Check sheet for the drawn part. Datum: minimum x, y, z corner. Units: mm. A direction names the side the tool comes from. Coordinates: 2 decimals unless noted, no trailing zeros. Write each loop counter-clockwise with the first axis right and the second up, starting at its lowest first coordinate (ties: lowest second). Pieces come first, ordered by that corner, then holes. Notation, with made-up numbers: (46.25, 32) -> (66.25, 32) arc R5 ccw to (66.25, 37) -> close; hole circle Ø6 at (-13, 50.25). An arc over 180 degrees is marked (long way). One line per question, with ' | ' between items.
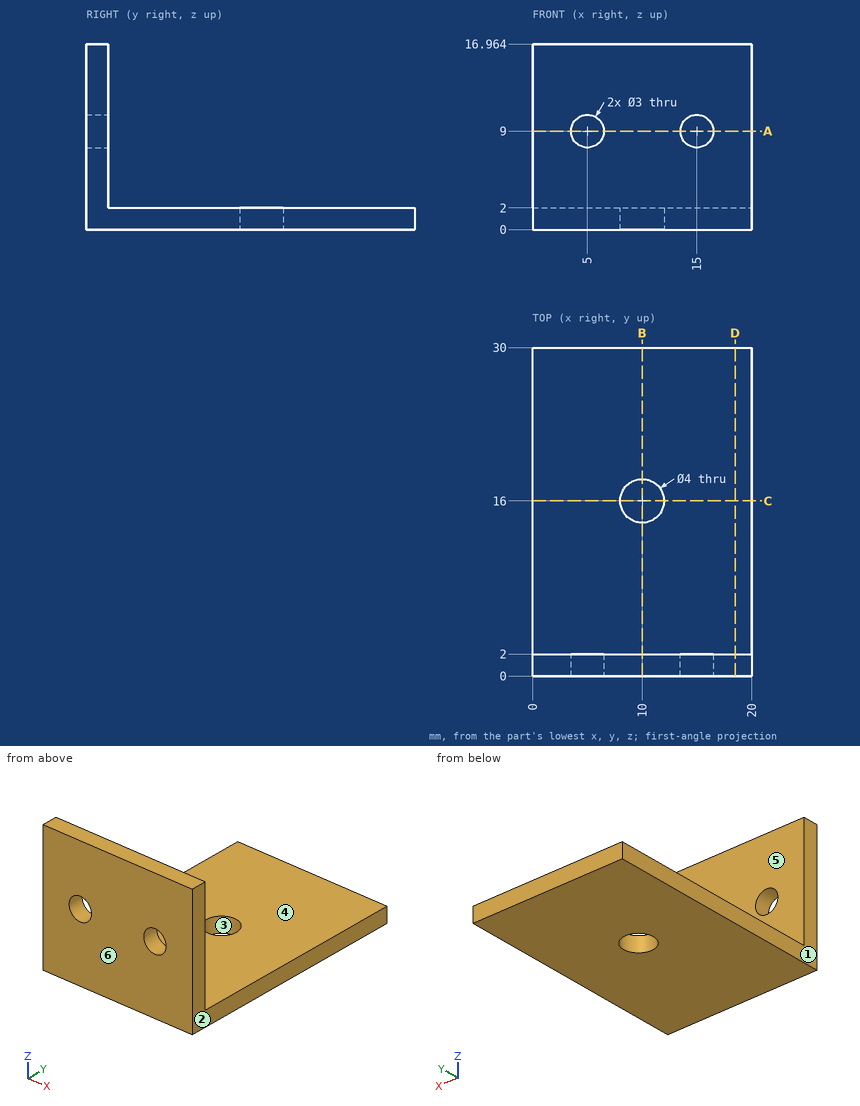
1. Cross-section at C-C on y = 16. Record the boundary of the cut face in (x, z).
Worked answers:
outline: (0, 0) -> (8, 0) -> (8, 2) -> (0, 2) -> close; (12, 0) -> (20, 0) -> (20, 2) -> (12, 2) -> close
2. Cross-section at A-A on z = 9. Record the boundary of the cut face in (x, y).
Worked answers:
outline: (0, 0) -> (3.5, 0) -> (3.5, 2) -> (0, 2) -> close; (6.5, 0) -> (13.5, 0) -> (13.5, 2) -> (6.5, 2) -> close; (16.5, 0) -> (20, 0) -> (20, 2) -> (16.5, 2) -> close
3. Cross-section at B-B on x = 10. Record the boundary of the cut face in (y, z).
Worked answers:
outline: (0, 0) -> (14, 0) -> (14, 2) -> (2, 2) -> (2, 16.96) -> (0, 16.96) -> close; (18, 0) -> (30, 0) -> (30, 2) -> (18, 2) -> close
4. Tool access check on the marked faces 5 and 6. Record the directions out of +Z, -Z, +X, -X, +Y, -Y that give a thin tool (end or side, any length) a straight path to the whole face; none if there is none.
Worked answers:
face 5: +Z, +X, -X, +Y | face 6: +Z, -Z, +X, -X, -Y
5. Mould release check, pull along X, two halves, no side actions. Record for the marked faces 1, 2, 3 and 4: released by +X, released by -X, zero draft, split by the parting line, or undercut.
Worked answers:
face 1: released by -X | face 2: released by +X | face 3: undercut | face 4: zero draft
6. Material ranges on line 1 (Z direction, x = 15, y = 0.55); line 2 (X direction, y = 0.5, z = 9); line 3 (Y direction, x = 10, z = 1.4), recorded low to high. Write a range as from..to.
Worked answers:
line 1: 0..7.5, 10.5..16.96 | line 2: 0..3.5, 6.5..13.5, 16.5..20 | line 3: 0..14, 18..30
7. Cross-section at D-D on x = 18.5. Record the boundary of the cut face in (y, z).
Worked answers:
outline: (0, 0) -> (30, 0) -> (30, 2) -> (2, 2) -> (2, 16.96) -> (0, 16.96) -> close
8. Go/stop test with flat-tipped pins: P1, Ø8, axis at x = 13, y = 21, coming from the +Z side; P2, Ø5, axis at x = 5, z = 9, coming from the +Y side. Record where each tip stops, or that it passes through.
Worked answers:
P1: z = 2 | P2: y = 2
